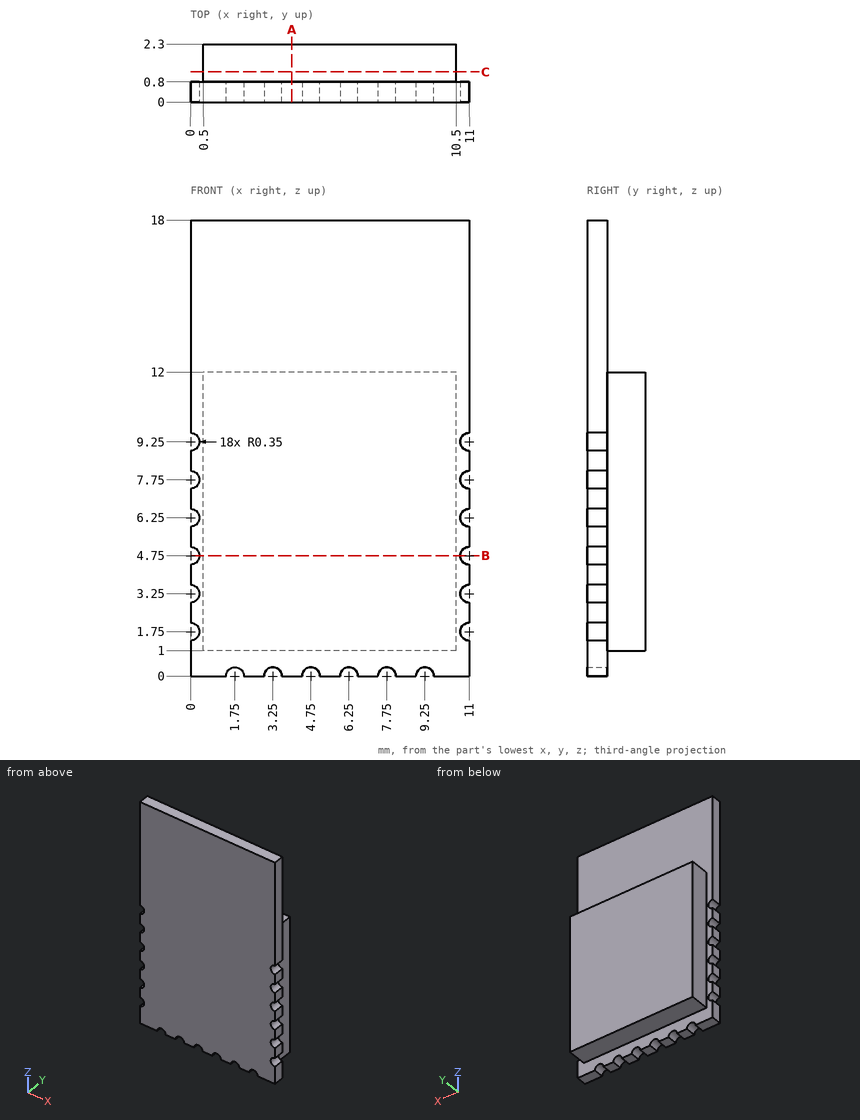
For this review, use the dimensioned drawing (mm, ordinates from the lowest corner) and the shaded views. Coordinates: 2 decimals unless noted, no trailing zeros. Order: outer loops, then holes, each group sorted by start corner. A loop starts at its lowest first (then second) coordinate and runs counter-clockwise, first axis right, second up. Notation, with made-up numbers: M 34,65 L 63,65 A20 ccw 63,96 Z; hole C 2.25,46 d11. An arc over 180 degrees is marked long. Answer as a JSON object with one key per item and string values. Group by question number.
1) Add section C-C, the plane y = 1.2. Write out the cut boundary in (x, z).
2) For pin 1 (1.2 mm diameter, centred on x = 4.5, y = 1.5, fed in from +Z); pin 2 (0.7 mm diameter, centred on x = 5, y = 1.5, fed in from -Z); pin 3 (0.7 mm diameter, centred on y = 1.5, z = 5, fed in from +X), all flat-tipped, find the tip position at first contact; note any pin that passes through.
3) Add section B-B, the plane z = 4.75. Write out the cut boundary in (x, y).
4) Wall thickness on L1, parallel to Z at x = 8, y = 1.65; L2, parallel to Y at x = 7.5, z = 15.5; L3, parallel to X at y = 1.55, z = 4.25: over which ranges is each line inside the solid? List them lowest first.
5) Add section A-A, the plane x = 4. Write out the cut boundary in (y, z).
Computed values:
{
 "1": {"outline": "M 0.5,1 L 10.5,1 L 10.5,12 L 0.5,12 Z"},
 "2": {"pin 1": "stops at z = 12", "pin 2": "stops at z = 1", "pin 3": "stops at x = 10.5"},
 "3": {"outline": "M 0.35,0 L 10.65,0 L 10.65,0.8 L 10.5,0.8 L 10.5,2.3 L 0.5,2.3 L 0.5,0.8 L 0.35,0.8 Z"},
 "4": {"L1": "z = 1 to 12", "L2": "y = 0 to 0.8", "L3": "x = 0.5 to 10.5"},
 "5": {"outline": "M 0,0 L 0.8,0 L 0.8,1 L 2.3,1 L 2.3,12 L 0.8,12 L 0.8,18 L 0,18 Z"}
}
